Geometry: final body of the model. Coordinates: model frame, mm. Coordinates: 2 decimals unless noted, no trailing zeros. Order: outer loops, then holes, each group sorted by start corner. A loop starts at its lowest first (then second) coordinate and runs counter-clockwise, first axis right, second up. Notation, with made-up numbers: M 56,38.5 L 75,38.5 A23 cw 75,70.5 Z; hole C 49.25,52.25 d4. An arc over 180 degrees is marked long. Use CSV: the item, a comma, the result in double quotes. Start each with the question number.
Q1. Section query D-D, the plane y = 47. Output: boundary loops of the cut face in (x, z), and give its area (3 significant figures).
Q2. Ray query, probe 1 along Y at (x, z) = (-23.5, 1.45); probe 2 along X at (y, z) = (84.5, 2.2); probe 3 along X at (y, z) = (64.5, 0.3). Return the intervals inside material, ascending.
Q3. Section query B-B, the plane y = 83.5. Output: boundary loops of the cut face in (x, z).
Q4. Section query A-A, the plane x = -14. Output: boundary loops of the cut face in (y, z), and give its area (3 significant figures).
Q5. Section query C-C, the plane z = 1.5. Output: boundary loops of the cut face in (x, y).
Q6. First-contact query: P1, Ø1, axis at x = 49, y = 81.5, coming from the -Z side; P2, Ø1.5, axis at x = 70, z = 2, coming from the +Y side. Flat tips, straight axial feed; report the tip coordinate or a pass-through.
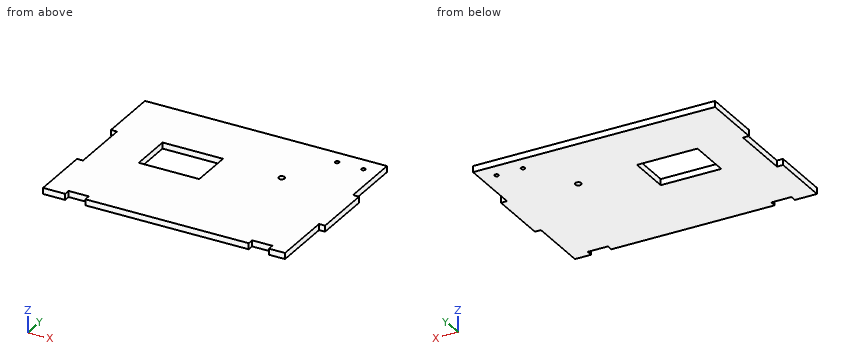
from build123d import *

# Parameters (mm, degrees)
MODEL_R             = 1
MODEL_R_2           = 1.5
MODEL_W             = 30
MODEL_H             = 21
BOSS_EXTRUDE1_DEPTH = 3


with BuildPart() as part:
    # Model → Boss-Extrude1 (new body)
    with BuildSketch(Plane.XY):
        Polygon((71.207281269, 100.913104874), (71.207281269, 70.913104874), (68.207281269, 70.913104874), (68.207281269, 40.913104874), (60.207281269, 40.913104874), (60.207281269, 43.913104874), (50.207281269, 43.913104874), (50.207281269, 40.913104874), (-30.792718731, 40.913104874), (-30.792718731, 43.913104874), (-40.792718731, 43.913104874), (-40.792718731, 40.913104874), (-51.792718731, 40.913104874), (-51.792718731, 70.913104874), (-48.792718731, 70.913104874), (-48.792718731, 100.913104874), (-51.792718731, 100.913104874), (-51.792718731, 130.913104874), (68.207281269, 130.913104874), (68.207281269, 100.913104874), align=None)
        with Locations((47.707281269, 123.413104874)):
            Circle(MODEL_R, mode=Mode.SUBTRACT)
        with Locations((60.707281269, 123.413104874)):
            Circle(MODEL_R, mode=Mode.SUBTRACT)
        with Locations((33.707281269, 99.413104874)):
            Circle(MODEL_R_2, mode=Mode.SUBTRACT)
        with Locations((-11.792718731, 91.413104874)):
            Rectangle(MODEL_W, MODEL_H, mode=Mode.SUBTRACT)
    extrude(amount=BOSS_EXTRUDE1_DEPTH)


solid = part.part
Responses:
1,outline,"M -51.79,0 L 68.21,0 L 68.21,3 L -51.79,3 Z"
1,area,"360 mm²"
2,probe 1,"y = 40.91 to 80.91, 101.91 to 130.91"
2,probe 2,"x = -48.79 to -26.79, 3.21 to 71.21"
2,probe 3,"x = -51.79 to 68.21"
3,outline,"M -48.79,0 L -26.79,0 L -26.79,3 L -48.79,3 Z; M 3.21,0 L 71.21,0 L 71.21,3 L 3.21,3 Z"
4,outline,"M 40.91,0 L 80.91,0 L 80.91,3 L 40.91,3 Z; M 101.91,0 L 130.91,0 L 130.91,3 L 101.91,3 Z"
4,area,"207 mm²"
5,outline,"M -51.79,40.91 L -40.79,40.91 L -40.79,43.91 L -30.79,43.91 L -30.79,40.91 L 50.21,40.91 L 50.21,43.91 L 60.21,43.91 L 60.21,40.91 L 68.21,40.91 L 68.21,70.91 L 71.21,70.91 L 71.21,100.91 L 68.21,100.91 L 68.21,130.91 L -51.79,130.91 L -51.79,100.91 L -48.79,100.91 L -48.79,70.91 L -51.79,70.91 Z; hole M -26.79,80.91 L 3.21,80.91 L 3.21,101.91 L -26.79,101.91 Z; hole C 33.71,99.41 d3; hole C 47.71,123.41 d2; hole C 60.71,123.41 d2"
6,P1,"stops at z = 0"
6,P2,"stops at y = 100.91"
